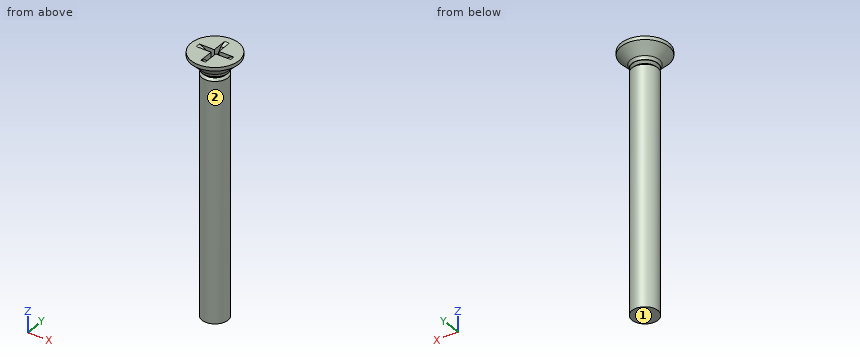
Autodesk Inventor part; units mm, degrees
ref_plane "MSC_PF1" through (0, 0, 0) normal (1, 0, 0) x (0, 1, 0)
ref_plane "MSC_PT1" through (0, 0, 0) normal (0, 0, -1) x (-1, 0, 0)
ref_plane "YZ Plane" through (0, 0, 0) normal (1, 0, 0) x (0, 1, 0)
sketch "Esquisse1" plane through (0, 0, 0) normal (0, 1, 0) x (-1, 0, 0)
  point P0 (0, 0)
sketch "Esquisse2" plane through (0, 0, 0) normal (0, 0, 1) x (1, 0, 0)
  point P0 (0, 0)
sketch "Esquisse3" plane through (0, 0, 0) normal (0, 0, 1) x (1, 0, 0)
  point P0 (0, 0)
sketch "Esquisse4" plane through (0, 0, 0) normal (0, 1, 0) x (-1, 0, 0)
  line L0 (-2.75, 0) -> (0, 0)
  line L1 (-2.75, -0.4) -> (-2.75, 0)
  line L2 (-1.5, -1.65) -> (-2.75, -0.4)
  line L3 (-1.5, -1.9) -> (-1.5, -1.65)
  line L4 (-1.25, -2.15) -> (-1.5, -1.9)
  line L5 (-1.5, -2.4) -> (-1.25, -2.15)
  line L6 (-1.5, -30) -> (-1.5, -2.4)
  line L7 (0, 0) -> (0, -30)
  line L8 (0, 3.3392) -> (0, -10.7) construction
  line L9 (0, 3.3392) -> (0, -10.7)
  line L10 (0, -36.6678) -> (0, 10.0071)
  line L11 (-1.5, -30) -> (0, -30)
  line L12 (0.55, 0) -> (-3.3, 0)
  dimension "d3" = 2.75
  dimension "d5" = 0.25
  dimension "d7" = 0.25
  dimension "d9" = 0.25
  dimension "d11" = 1.65
  dimension "d13" = 135
  dimension "d17" = 1.25
  dimension "d19" = 0
  dimension "d51" = 1.5
  dimension "d52" = 30
revolve "Révolution1" add sketch "Esquisse4" angle 360 about axis through (0, 0, 3.3392) along (0, 0, -1)
sketch "Esquisse5" plane through (0, 0, 0) normal (0, 1, 0) x (-1, 0, 0)
  line L0 (-1.6, 0) -> (0, 0)
  line L1 (-0.2667, -1.5) -> (-1.6, 0)
  line L2 (0, -1.5) -> (-0.2667, -1.5)
  line L3 (0, 0) -> (0, -1.5)
  line L4 (-1.5, -1.65) -> (1.5, -1.65) construction
  line L5 (-2.75, 0) -> (2.75, 0)
  line L6 (0, -1.98) -> (0, 0.33)
  dimension "d22" = 1.6
  dimension "d24" = 0.2667
  dimension "d26" = 1.5
extrude "Extrusion1" cut sketch "Esquisse5" along normal mid plane 0.5333
pattern_circular "RéseauPolaire1" count 4 over 360 about axis through (0, 0, 0) along (0, 0, 1) of "Extrusion1"
sketch "Esquisse7" plane through (0, 0, 0) normal (0, 1, 0) x (-1, 0, 0)
  line L0 (0, -0.825) -> (-2, 0)
  line L1 (0, 0) -> (0, -0.825)
  line L2 (-2, 0) -> (0, 0)
  line L3 (-1.5, -1.65) -> (1.5, -1.65) construction
  line L4 (0, -1.98) -> (0, 0.33)
  line L5 (-2.75, 0) -> (2.75, 0)
  dimension "d33" = 2
  dimension "d35" = 0.825
extrude "Extrusion2" cut sketch "Esquisse7" along normal mid plane 0.5333
pattern_circular "RéseauPolaire2" count 4 over 360 about axis through (0, 0, 0) along (0, 0, 1) of "Extrusion2"
fillet "Congé1" radius 0.5 1 edges at (-1.5, 0, -1.65)
thread "Filetage1"
ref_plane "MSC_PF1" through (0, 0, 0) normal (1, 0, 0) x (0, 1, 0)
ref_plane "MSC_PT1" through (0, 0, 0) normal (0, 0, -1) x (-1, 0, 0)
equation "\"d3\" = 0.5 * Dh"
equation "\"d5\" = msp_x"
equation "\"d7\" = ParA"
equation "\"d9\" = msp_x"
equation "\"d11\" = ParK"
equation "\"d17\" = 0.5 * msp_mdtds"
equation "\"d51\" = 0.5 * NND"
equation "\"d52\" = NLG"
equation "\"d22\" = 0.5 * M"
equation "\"d24\" = 0.0833333 * M"
equation "\"d26\" = 0.909091 * ParK"
equation "\"d27\" = 0.166667 * M"
equation "\"d33\" = 0.625 * M"
equation "\"d35\" = 0.5 * ParK"
equation "\"d36\" = 0.166667 * M"
equation "\"d41\" = 2 * msp_x"
equation "\"PTC\" = 0.5"
equation "\"NLG\" = 30"
equation "\"ParK\" = 1.65"
equation "\"NND\" = 3"
equation "\"M\" = 3.2"
equation "\"msp_mdtds\" = NND - PTC"
equation "\"Dh\" = 5.5"
equation "\"msp_x\" = 0.5 * PTC"
equation "\"ParA\" = 0.5 * PTC"
equation "\"r\" = 0.8"
equation "\"THREADDIA\" = NND"
equation "\"TEMPLATE\" = 1.2345"
properties part number "NF EN ISO 7046-2 H - M3x30 - 8.8 - H1" material "Acier inoxydable 440C"
The listing builds one solid part. Answer for the finished solid, in the listing's coordinates (mm). Face numbers are marked on the shaded views. A direction names the side the tool comes from. Round coordinates to 2 decimals unless told otherwise and drop trailing zeros. Order: outer loops, then holes, each group sorted by start corner. A loop starts at its lowest first (then second) coordinate and runs counter-clockwise, first axis right, second up. Notation, with made-up numbers: M 72.5,-9.75 L 76.5,-9.75 A29 ccw 76.5,21.25 Z; hole C 36.25,80.25 d4. An arc over 180 degrees is marked long. Answer in a Markdown table with one row per item. Add a question column.
1) Which of the six approach directions +Z, -Z, +X, -X, +Y, -Y give full straight-line access (tool end or side, diameter ignored) to the marked faces 1 and 2?
2) Flat-ended cylindrical pins translate along their axes: pin 1 Ø2 at (y, z) = (-1, -11.5) entering from -X; pin 2 Ø1.7 at (y, z) = (1.5, -1) entering from -X; pin 3 Ø0.8 at (y, z) = (-1, -0.5) entering from +X. Find the tip coordinate at first contact, or state that the pin passes through.
3) The part is cut by section A-A on z = -20.5. Determine the outline of the cut face in (x, y).
4) Consider line 1 along X through (y, z) = (0.6, -9); line 2 along Z through (x, y) = (1.3, 0.4); line 3 along Z through (x, y) = (-1.15, -2.4). Determine where each line is inside the solid, lowest interval first. Write a range as from..to.
Findings below:
| question | item | result |
|---|---|---|
| 1 | face 1 | -Z, +X, -X, +Y, -Y |
| 1 | face 2 | -Z |
| 2 | pin 1 | stops at x = -1.5 |
| 2 | pin 2 | stops at x = -2.6 |
| 2 | pin 3 | stops at x = 2.68 |
| 3 | outline | C 0,0 d3 |
| 4 | line 1 | x = -1.37..1.37 |
| 4 | line 2 | z = -30..-2.26, -2.04..0 |
| 4 | line 3 | z = -0.49..0 |
